Build history of the part. All positions in model axes, mm. Face numbers are marked on the shaded views. A direction names the side the tool comes from. Give positions to 0.01 mm unless a question says otherwise; leave off trailing zeros. Loops run counter-clockwise (first coordinate to the right, second up) from the corner with the lowest first, then second, coordinate; pieces in that order, holes last. Notation, with made-up numbers: (-13, 1) -> (10, 1) arc R26 cw to (10, 17) -> close; hole circle Ø4 at (3, 26.5). An arc over 180 degrees is marked (long way). One line per question, with ' | ' between items. Start each with the question number.
(1) Slice it at C-C, the plane x = 21. Write the cut outline in (y, z).
(2) 3-axis set-ups, long thin cutter, end or side, ignore diameter. For the marked faces 1, 2 and 3: which of +Z, -Z, +X, -X, +Y, -Y reach the whole face in a straight line?
(3) Flat gauge pins, fed straight in: pin 1 Ø5.5 at (y, z) = (5, -15.5) entering from -X; pin 2 Ø1 at (x, y) = (11.5, 8.5) entering from +Z; pin 3 Ø3 at (x, y) = (15, 12.5) entering from +Z; pin 4 Ø5.5 at (x, y) = (12.5, 9) entering from -Z. Where does each tip first touch, or does it go through?
(4) Drill centre lines: L1, parallel to Z at x = 12.5, y = 16.6; L2, parallel to Z at x = 9, y = 16.75; L3, parallel to Z at x = 8.5, y = 5. Where is each one in solid material? Low to high. Write a range as from..to.
(5) Slice it at A-A, the plane x = 12.5. Write the cut outline in (y, z).
(6) Slice it at B-B, the plane y = 6.75. Write the cut outline in (x, z), then the cut area to 4 significant figures.
Autodesk Inventor part; units mm, degrees
ref_plane "Work Plane1" through (0, 13.1625, 0) normal (0, 1, 0) x (1, 0, 0)
ref_plane "YZ Plane" through (0, 0, 0) normal (1, 0, 0) x (0, 1, 0)
ref_plane "XZ Plane" through (0, 0, 0) normal (0, 1, 0) x (-1, 0, 0)
sketch "Sketch1" plane through (0, 0, 0) normal (1, 0, 0) x (0, 1, 0)
  line L0 (0, 0) -> (9.5813, 0)
  line L1 (9.5813, 0) -> (9.5812, 23)
  line L2 (7.5812, 25) -> (0, 25)
  line L3 (0, 25) -> (0, 0)
  line L4 (9.5812, 23) -> (7.5812, 25)
  line L5 (0, 0) -> (19.1625, 0)
  line L6 (19.1625, 0) -> (19.1625, -20)
  line L7 (19.1625, -20) -> (15, -20)
  line L8 (0, -5) -> (0, 0)
  line L9 (19.1625, -20) -> (11.1625, -20)
  line L10 (15, -20) -> (0, -5)
  point P0 (9.5812, 25)
  point P1 (0, -20)
  dimension "d0" = 9.5813
  dimension "d1" = 25
  dimension "d2" = 2
  dimension "d3" = 2
  dimension "d4" = 20
  dimension "d5" = 19.1625
  dimension "d8" = 15
  dimension "d9" = 15
extrude "Extrusion1" add sketch "Sketch1" along normal blind 25
ref_plane "Work Plane1" through (0, 13.1625, 0) normal (0, 1, 0) x (1, 0, 0)
sketch "Sketch2" plane through (0, 13.1625, 0) normal (0, 1, 0) x (1, 0, 0)
  line L0 (20, 30.2149) -> (5, 30.2149)
  line L1 (5, 30.2149) -> (5, 7)
  line L2 (5, 7) -> (20, 7)
  line L3 (20, 7) -> (20, 30.2149)
  line L4 (25, 5) -> (25, 20)
  line L5 (0, 5) -> (0, 20)
  line L6 (0, 0) -> (25, 0)
  dimension "d13" = 5
  dimension "d14" = 5
  dimension "d15" = 7
extrude "Extrusion2" cut sketch "Sketch2" against normal blind 25
sketch "Sketch3" plane through (0, 13.1625, 0) normal (0, -1, 0) x (1, 0, 0)
  circle A0 centre (12.5, -12.5813) radius 2
  line L0 (20, -7) -> (20, -18.1625)
  point P0 (0, 0)
  point P1 (20, -12.5813)
  dimension "d18" = 4
  dimension "d19" = 0
extrude "Extrusion3" cut sketch "Sketch3" against normal blind 25
chamfer "Chamfer1" distance 2 angle 45 1 edges at (10.5, 13.1625, -12.5813)
properties part number "front wall bkt"
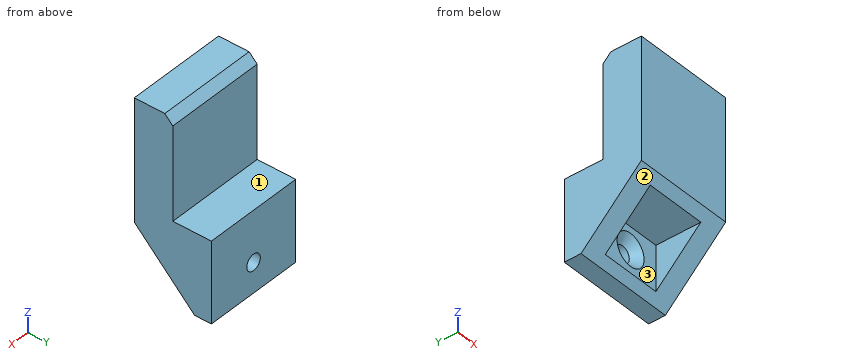
Final values:
1) outline: (0, -5) -> (15, -20) -> (19.16, -20) -> (19.16, 0) -> (9.58, 0) -> (9.58, 23) -> (7.58, 25) -> (0, 25) -> close
2) face 1: +Z, +X, -X, +Y | face 2: -Z, +X, -X, -Y | face 3: -Z, -Y
3) pin 1: through | pin 2: z = 24.58 | pin 3: z = 0 | pin 4: z = -7
4) L1: -20..-14.58, -10.58..0 | L2: -20..0 | L3: -7..25
5) outline: (0, -5) -> (2, -7) -> (13.16, -7) -> (13.16, -8.58) -> (15.16, -10.58) -> (19.16, -10.58) -> (19.16, 0) -> (9.58, 0) -> (9.58, 23) -> (7.58, 25) -> (0, 25) -> close; (13.16, -18.16) -> (15, -20) -> (19.16, -20) -> (19.16, -14.58) -> (15.16, -14.58) -> (13.16, -16.58) -> close
6) outline: (0, -11.75) -> (5, -11.75) -> (5, -7) -> (20, -7) -> (20, -11.75) -> (25, -11.75) -> (25, 25) -> (0, 25) -> close | area: 847.5 mm2
